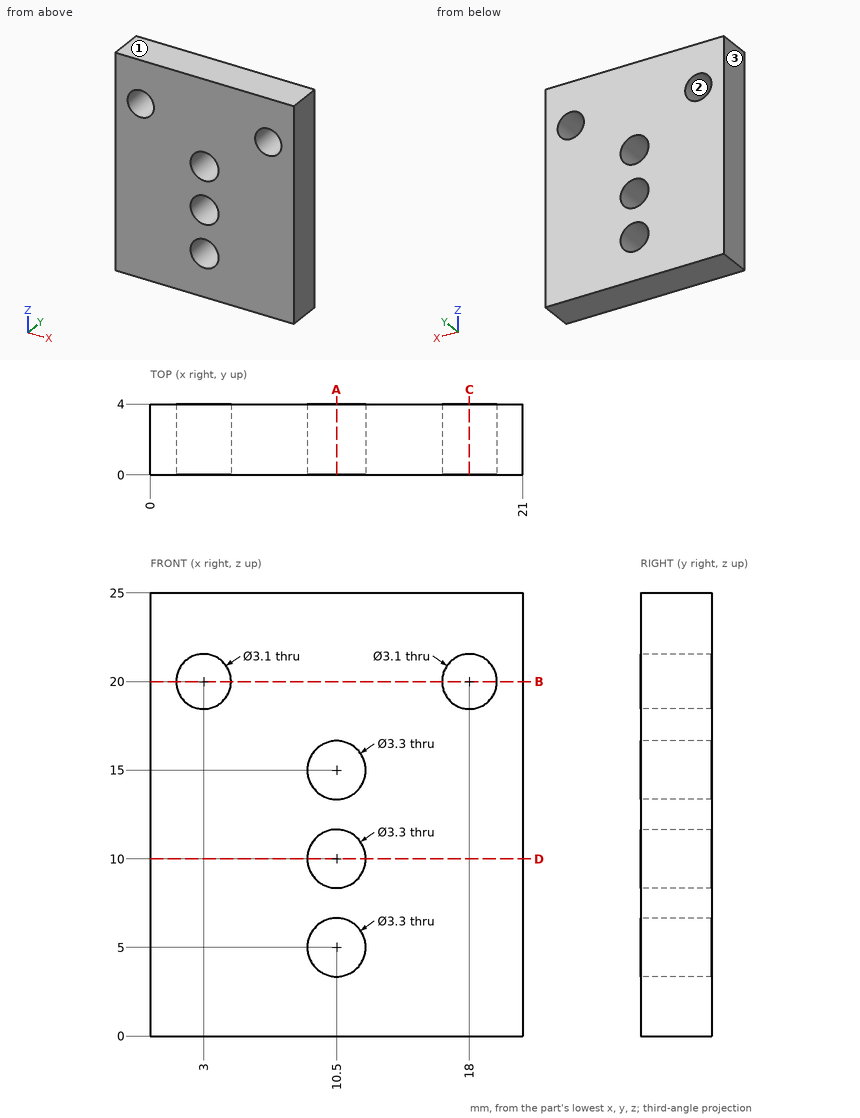
Geometry: see drawing. Coordinates: mm, zero at the bounding-box minimum. Round coordinates to 2 decimals unless told otherwise and drop trailing zeros. Loops run counter-clockwise (first coordinate to the right, second up) from the corner with the lowest first, then second, coordinate; pieces in that order, holes last. Notation, with made-up numbers: (-15.5, 70) - (-5.5, 70) arc R17 ccw to (-5.5, 86) - close; hole circle Ø1 at (83.5, 0.5). An arc over 180 degrees is marked (long way). One line per item, written item: value. Start each with the question number.
(1) Ray query, line 1 (X direction, y = 1.95, z = 20); line 2 (X direction, y = 0.9, z = 5); line 3 (Z direction, x = 18, y = 1.9). Return the intervals inside material, ascending. Write a range as [from, to].
(2) Contact query for flat-ended pins moving along their axis: P1, Ø4, axis at x = 18, z = 20, coming from the -Y side; P2, Ø1.9, axis at x = 3, z = 20, coming from the -Y side. Output: stop coordinate, or through.
(3) Section C-C, the plane x = 18. Return loops of the section in (y, z).
(4) Section B-B, the plane z = 20. Return loops of the section in (x, y).
(5) Draft query along X for the marked faces 1, 2 and 3. Return one class per face: +X half, -X half, draft (parallel to the pull), parting line (faces both ways), or undercut.
(6) Section D-D, the plane z = 10. Return loops of the section in (x, y), plus the area to 3 significant figures.
(7) Section A-A, the plane x = 10.5. Return loops of the section in (y, z).
Results below:
1. line 1: [0, 1.45], [4.55, 16.45], [19.55, 21]
1. line 2: [0, 8.85], [12.15, 21]
1. line 3: [0, 18.45], [21.55, 25]
2. P1: y = 0
2. P2: through
3. outline: (0, 0) - (4, 0) - (4, 18.45) - (0, 18.45) - close; (0, 21.55) - (4, 21.55) - (4, 25) - (0, 25) - close
4. outline: (0, 0) - (1.45, 0) - (1.45, 4) - (0, 4) - close; (4.55, 0) - (16.45, 0) - (16.45, 4) - (4.55, 4) - close; (19.55, 0) - (21, 0) - (21, 4) - (19.55, 4) - close
5. face 1: draft
5. face 2: undercut
5. face 3: -X half
6. outline: (0, 0) - (8.85, 0) - (8.85, 4) - (0, 4) - close; (12.15, 0) - (21, 0) - (21, 4) - (12.15, 4) - close
6. area: 70.8 mm^2
7. outline: (0, 0) - (4, 0) - (4, 3.35) - (0, 3.35) - close; (0, 6.65) - (4, 6.65) - (4, 8.35) - (0, 8.35) - close; (0, 11.65) - (4, 11.65) - (4, 13.35) - (0, 13.35) - close; (0, 16.65) - (4, 16.65) - (4, 25) - (0, 25) - close
